Here's how the part is built. I have some questions about the finished solid (model axes, mm). Face numbers are marked on the shaded views. A direction names the side the tool comes from. Round coordinates to 2 decimals unless told otherwise and drop trailing zeros. Order: outer loops, then holes, each group sorted by start corner. A loop starts at its lowest first (then second) coordinate and runs counter-clockwise, first axis right, second up. Notation, with made-up numbers: M 28,77.5 L 55,77.5 A22 cw 55,85.5 Z; hole C 6.25,61.5 d8. An arc over 180 degrees is marked long. Write item = value, one per line. Start each with the question number.
Item 1: Please list where these lines run through material, in increasing order: L1, parallel to X at y = 131, z = -30; L2, parallel to Y at x = -54, z = 14; L3, parallel to Y at x = 41, z = 16.
Item 2: I want a section at B-B, the plane z = 68. List the corners of the cut face in (x, y) for me, plus the area to 3 significant figures.
Item 3: I'm going to push flat-ended pins straight in: P1, Ø16, axis at x = 38, z = -65.82, coming from the +Y side; P2, Ø12, axis at y = 23.5, z = 5, coming from the -X side; P3, Ø8, axis at y = 118, z = 39.5, coming from the -X side; P4, Ø12, axis at x = -9.5, y = 112, coming from the +Z side. Where does each tip first touch, or does it pass through?
Item 4: I want a section at C-C, the plane y = 15. List the corners of the cut face in (x, z) for me, plus the area to 3 significant figures.
Item 5: I want a section at D-D, the plane y = 132. State how many separate pieces and enclosed holes the cut face has, plus the area to 3 significant figures.
Item 6: For the marked faces 4, 5 and 6, which set-ups out of +Z, -Z, +X, -X, +Y, -Y let a thin tool reach every point of the face, with its end or its side?
Item 7: We'd pull the mould along Z, two halves only. Please class the marked faces 1, 2 and 3: pulls with the +Z half, pulls with the -Z half, needs draft (parallel to the pull), parting line crosses it, or undercut.
```python
from build123d import *

# Parameters (mm, degrees)
HOLE1_D           = 20
CIRPATTERN1_COUNT = 6
CIRPATTERN2_COUNT = 6


with BuildPart() as part:
    # Sketch1 → Revolve1 (revolve)
    with BuildSketch(Plane.XY, mode=Mode.PRIVATE) as revolve1_sk:
        Polygon((22, 0), (44, 110), (54, 110), (54, 120), (103, 120), (103, 136), (51, 136), (51, 141), (0, 141), (0, 0), align=None)
    revolve(revolve1_sk.sketch.rotate(Axis((0, 141, 0), (0, -1, 0)), 180), axis=Axis((0, 141, 0), (0, -1, 0)))

    # Sketch2 → Cut-Revolve1 (revolve, cut)
    with BuildSketch(Plane.XY, mode=Mode.PRIVATE) as cut_revolve1_sk:
        Polygon((0, 0), (11.414348642, 0), (11.414348642, 38), (16, 42.585651358), (16, 54.752962034), (11, 58), (11, 75), (22, 86), (22, 141), (0, 141), align=None)
    revolve(cut_revolve1_sk.sketch.rotate(Axis((0, 141, 0), (0, -1, 0)), 180), axis=Axis((0, 141, 0), (0, -1, 0)), mode=Mode.SUBTRACT)

    # Hole1 (through all)
    with Locations(Plane(origin=(0, 136, 0), x_dir=(1, 0, 0), z_dir=(0, 1, 0))):
        with Locations((76, 0)):
            hole1 = Hole(HOLE1_D / 2)

    # CirPattern1: Hole1 ×6 about axis
    cirpattern1_axis = Axis((0, 0, 0), (0, 1, 0))
    for i in range(1, CIRPATTERN1_COUNT):
        add(hole1.rotate(cirpattern1_axis, i * 360 / CIRPATTERN1_COUNT), mode=Mode.SUBTRACT)

    # Sketch9 → M10x1.0 Tapped Hole5 (revolve, cut)
    with BuildSketch(Plane(origin=(38, 141, 0), x_dir=(0, 0, 1), z_dir=(1, 0, 0))):
        Polygon((0, 0), (0, 17.703872786), (4.5, 15), (4.5, 0.525), (5.025, 0), align=None)
    m10x1_0_tapped_hole5 = revolve(axis=Axis((38, 147.35, 0), (0, -1, 0)), mode=Mode.SUBTRACT)

    # CirPattern2: M10x1.0 Tapped Hole5 ×6 about axis
    cirpattern2_axis = Axis((0, 0, 0), (0, 1, 0))
    for i in range(1, CIRPATTERN2_COUNT):
        add(m10x1_0_tapped_hole5.rotate(cirpattern2_axis, i * 360 / CIRPATTERN2_COUNT), mode=Mode.SUBTRACT)


solid = part.part
```
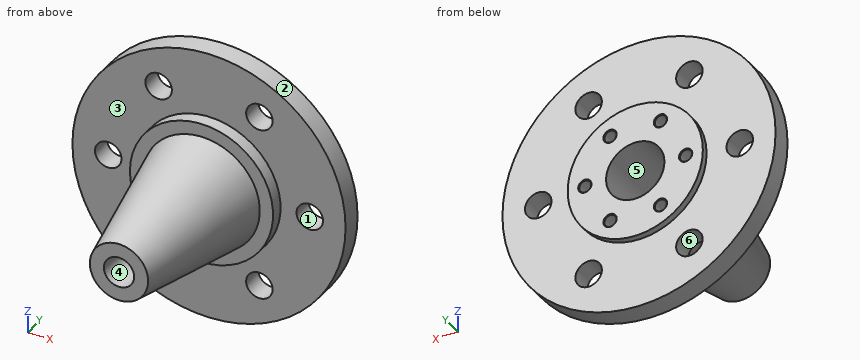
Filled in:
q1.L1 = -98.53 to -22.43, -15.57 to 15.57, 22.43 to 98.53
q1.L2 = 120 to 136
q1.L3 = 110 to 141
q2.outline = M -77.36,120 L -47.76,120 L -47.76,136 L -77.36,136 Z; M -28.24,120 L 28.24,120 L 28.24,136 L -28.24,136 Z; M 47.76,120 L 77.36,120 L 77.36,136 L 47.76,136 Z
q2.area = 1,850 mm^2
q3.P1 = through
q3.P2 = -27.68
q3.P3 = -96.49
q3.P4 = 53.89
q4.outline = C 0,0 d50; hole C 0,0 d22.83
q4.area = 1,550 mm^2
q5.separate_pieces = 1
q5.enclosed_holes = 13
q5.area = 29,500 mm^2
q6.face_4 = -Y
q6.face_5 = +Y
q6.face_6 = +Y, -Y
q7.face_1 = undercut
q7.face_2 = parting line crosses it
q7.face_3 = needs draft
